Verification items for the finished model (mm, model axes). A direction names the side the tool comes from. Give positions to 0.01 mm unless a question says otherwise; leave off trailing zeros. Order: outer loops, then holes, each group sorted by start corner. A loop starts at its lowest first (then second) coordinate and runs counter-clockwise, first axis right, second up.
(1) Access from +Z, -Z, +X, -X, +Y, -Y to the whole of each face (thin tool, end or side, straight path). Record for faces 1 (the face through (0, -46, 1)), 2 (the face through (47, 0, 1)), 3 (the face through (78.74, -40, 1)).
(2) Sectioned sample at A-A on z = 1.75. Record the cut outline in (x, y) (3 decimals), plus the area to 3 significant figures.
(3) Sectioned sample at C-C on x = 59. Record the cut outline in (y, z), plus the area to 3 significant figures.
(4) Gauge pin test, flat ends, axial feed: pin 1 (0.8 mm diameter, centred on y = -54, z = 1.5, fed in from -X); pin 2 (8 mm diameter, centred on x = 0, y = 0, fed in from +Z); pin 3 (0.8 mm diameter, centred on x = 58.5, z = 1.5, fed in from +Y). Record the tip position at first contact, or that the pin passes through.
(5) Sectioned sample at D-D on y = -30. Record the cut outline in (x, z).
(6) Sectioned sample at B-B on x = 1.5. Record the cut outline in (y, z), plus the area to 3 significant figures.
(7) Scan lines: L1, parallel to X at y = -69, z = 1.95; L2, parallel to Y at x = 27.5, z = 1.4; L3, parallel to X at y = -2, z = 2.05. Record each from-to range of solid material in increasing order.
(8) Mould release check, pull along X, two halves, no side actions. Record for faces 4 (the face through (11.554, 0.963, 1.288)), 5 (the face through (34, -34, 2.54)), 6 (the face through (-0.91, -11.63, 1.29)), 7 (the face through (-0.96, -4.34, 1.25)): pulls with the +X half, pulls with the -X half, needs draft (parallel to the pull), parting line crosses it, or undercut.
```python
from build123d import *

# Parameters (mm, degrees)
SKETCH1_R           = 4.445
BOSS_EXTRUDE1_DEPTH = 2.54
FILLET1_R           = 5.08


with BuildPart() as part:
    # Sketch1 → Boss-Extrude1 (new body)
    with BuildSketch(Plane.XY):
        with BuildLine():
            Line((0, -10.3124), (0, -78.74))
            Line((0, -78.74), (78.74, -78.74))
            Line((78.74, -78.74), (78.74, 0))
            Line((78.74, 0), (10.3124, 0))
            ThreePointArc((10.3124, 0), (-7.29196797, 7.29196797), (0, -10.3124))
        make_face()
        Circle(SKETCH1_R, mode=Mode.SUBTRACT)
    extrude(amount=BOSS_EXTRUDE1_DEPTH)

    # Fillet1
    fillet1_edges = [part.edges().sort_by_distance(p)[0] for p in [
        (0, -10.3124, 1.27),
        (10.3124, 0, 1.27),
    ]]
    fillet(fillet1_edges, radius=FILLET1_R)


solid = part.part
```
Ans:
1. face 1: +Z, -Z, -X, -Y
1. face 2: +Z, -Z, +X, +Y
1. face 3: +Z, -Z, +X, +Y, -Y
2. outline: (-3.403, -9.735) arc R5.08 cw to (0, -14.53) - (0, -78.74) - (78.74, -78.74) - (78.74, 0) - (14.53, 0) arc R5.08 cw to (9.735, 3.403) arc R10.312 ccw (long way) to start; hole circle Ø8.89 at (0, 0)
2. area: 6,390 mm2
3. outline: (-78.74, 0) - (0, 0) - (0, 2.54) - (-78.74, 2.54) - close
3. area: 200 mm2
4. pin 1: stops at x = 0
4. pin 2: passes through
4. pin 3: stops at y = 0
5. outline: (0, 0) - (78.74, 0) - (78.74, 2.54) - (0, 2.54) - close
6. outline: (-78.74, 0) - (-4.18, 0) - (-4.18, 2.54) - (-78.74, 2.54) - close; (4.18, 0) - (10.2, 0) - (10.2, 2.54) - (4.18, 2.54) - close
6. area: 205 mm2
7. L1: x = 0 to 78.74
7. L2: y = -78.74 to 0
7. L3: x = -10.12 to -3.97, 3.97 to 78.74
8. face 4: pulls with the +X half
8. face 5: needs draft
8. face 6: pulls with the -X half
8. face 7: undercut
